Design review of the part built by this model. Coordinates are the model's own, in mm. Face numbers are marked on the shaded views. A direction names the side the tool comes from. Coordinates: 2 decimals unless noted, no trailing zeros. Loops run counter-clockwise (first coordinate to the right, second up) from the corner with the lowest first, then second, coordinate; pieces in that order, holes last. Notation, with made-up numbers: M 64,-19 L 78,-19 A9 ccw 78,-11 Z; hole C -20,50 d9. An arc over 180 degrees is marked long. Answer as a JSON object with one key per item and string values. Group by question number.
1. Consider section B-B (z = 23.5). State the section outline as (x, y) points, then the cut area to 3 significant figures.
2. To check wall thickness, follow probe 1 along Z at (x, y) = (11, 18.5) (1 decimal); probe 2 along X at (y, z) = (7.5, 32); probe 3 along Z at (x, y) = (-17.5, 2) (3 decimals). State the ranges of each line that lie inside material, in increasing order.
3. Consider section A-A (x = 0). State the section outline as (y, z) points (1 decimal), then the cut area to 3 significant figures.
4. Draft analysis for pull direction Z (two halves, no side actions). For the marked faces 1, 2 and 3, state which applies: +Z half, -Z half, draft (parallel to the pull), parting line (faces both ways), or undercut.
5. Insertion check: pin 1 (17.5 mm diameter, centred on x = -0.5, z = -31.5, fed in from +Y); pin 2 (23 mm diameter, centred on x = -0.5, y = 19, fed in from +Z); pin 3 (4 mm diameter, centred on y = 13.5, z = 30, fed in from +X). Each pin has a flat end and moves straight along its axis. Give the tip position at first contact, or say it passes through.
6. Machinability: for the marked faces 4, 5 and 6, which of the approach directions +Z, -Z, +X, -X, +Y, -Y give a long, thin tool a straight path to every point of the face, cutting with its end or side? Answer none if there is none.
7. Consider section D-D (z = 31.5). State the section outline as (x, y) points, then the cut area to 3 significant figures.
8. Consider section C-C (x = 9.5). State the section outline as (y, z) points (3 decimals).
Autodesk Inventor part; units mm, degrees
ref_plane "YZ Plane" through (0, 0, 0) normal (1, 0, 0) x (0, 1, 0)
ref_plane "XZ Plane" through (0, 0, 0) normal (0, 1, 0) x (-1, 0, 0)
ref_plane "XY Plane" through (0, 0, 0) normal (0, 0, 1) x (1, 0, 0)
sketch "Sketch2" plane through (0, 0, 0) normal (0, 1, 0) x (-1, 0, 0)
  line L0 (-26.1, 38) -> (26.1, 38)
  line L1 (26.1, 38) -> (26.1, -38)
  line L2 (26.1, -38) -> (-26.1, -38)
  line L3 (-26.1, -38) -> (-26.1, 38)
  line L4 (-26.1, 38) -> (26.1, -38) construction
  line L5 (26.1, 38) -> (-26.1, -38) construction
  line L6 (26.1, 22.085) -> (-26.1, 22.085)
  line L7 (-26.1, 22.085) -> (-26.1, -22.085)
  line L8 (-26.1, -22.085) -> (26.1, -22.085)
  line L9 (26.1, -22.085) -> (26.1, 22.085)
  line L10 (26.1, 22.085) -> (-26.1, -22.085) construction
  line L11 (-26.1, 22.085) -> (26.1, -22.085) construction
  line L12 (26.1, 38) -> (-26.1, 22.085) construction
  circle A0 centre (0, 30.0425) radius 5
  circle A1 centre (11, 30.0425) radius 5
  circle A2 centre (-11, 30.0425) radius 5
  point P0 (0, 0)
  dimension "d0" = 52.2
  dimension "d1" = 76
  dimension "d2" = 44.17
  dimension "OutCableDia" = 10
  dimension "d9" = 10
  dimension "d10" = 10
  dimension "d11" = 11
  dimension "d12" = 11
extrude "Extrusion1" add sketch "Sketch2" against normal blind 18 contours L0 L1 L6 L3 | L6 L1 L8 L3 | L8 L1 L2 L3 | A0 | A1 | A2
extrude "Extrusion2" add sketch "Sketch2" along normal blind 29 contours L6 L1 L8 L3
extrude "Extrusion3" add sketch "Sketch2" along normal blind 29 contours A0 | A1 | A2
equation "\"d9\" = OutCableDia"
equation "\"d10\" = OutCableDia"
properties part number "HobbyWing EZRUN 150A Pro 2"
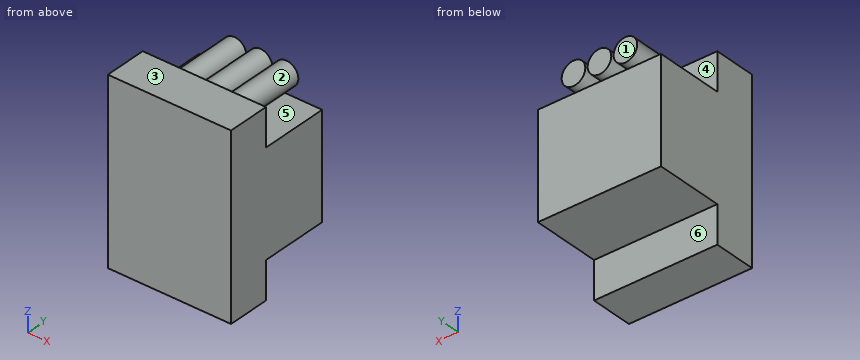
Findings below:
{
 "1": {"outline": "M -26.1,-18 L 26.1,-18 L 26.1,0 L -26.1,0 Z", "area": "940 mm^2"},
 "2": {"probe 1": "z = -22.1 to 22.1, 25 to 35", "probe 2": "x = -15.6 to -6.4, -4.6 to 4.6, 6.4 to 15.6", "probe 3": "z = -22.085 to 22.085"},
 "3": {"outline": "M -18,-38 L 0,-38 L 0,-22.1 L 29,-22.1 L 29,22.1 L 0,22.1 L 0,25 L 29,25 L 29,35 L 0,35 L 0,38 L -18,38 Z", "area": "2,940 mm^2"},
 "4": {"face 1": "draft", "face 2": "undercut", "face 3": "+Z half"},
 "5": {"pin 1": "stops at y = 0", "pin 2": "stops at z = 35.04", "pin 3": "stops at x = 16"},
 "6": {"face 4": "+Y", "face 5": "+X, -X, +Y", "face 6": "-Z, +X, -X, +Y"},
 "7": {"outline": "M -26.1,-18 L 26.1,-18 L 26.1,0 L 15.78,0 L 15.78,29 L 6.22,29 L 6.22,0 L 4.78,0 L 4.78,29 L -4.78,29 L -4.78,0 L -6.22,0 L -6.22,29 L -15.78,29 L -15.78,0 L -26.1,0 Z", "area": "1,770 mm^2"},
 "8": {"outline": "M -18,-38 L 0,-38 L 0,-22.085 L 29,-22.085 L 29,22.085 L 0,22.085 L 0,25.273 L 29,25.273 L 29,34.812 L 0,34.812 L 0,38 L -18,38 Z"}
}
